from build123d import *

# Parameters (mm, degrees)
F0_R     = 12.7
F1_DEPTH = 25.4
F2_W     = 88.9
F2_H     = 50.8
F3_DEPTH = 50.8
F5_DEPTH = 88.9
F7_DEPTH = 75.946
F8_R     = 12.7
F9_DEPTH = 112.776


# Not quite as in the source:
# - a feature names something its author has since deleted; it is built from what else it names


with BuildPart() as f1:
    # F0 (on Top) → F1 (new body)
    with BuildSketch(Plane.XY):
        with BuildLine():
            Line((-63.5, -31.75), (63.5, -31.75))
            ThreePointArc((63.5, -31.75), (95.25, 0), (63.5, 31.75))
            Line((63.5, 31.75), (-63.5, 31.75))
            ThreePointArc((-63.5, 31.75), (-95.25, 0), (-63.5, -31.75))
        make_face()
        with Locations((-63.5, 0)):
            Circle(F0_R, mode=Mode.SUBTRACT)
        with Locations((63.5, 0)):
            Circle(F0_R, mode=Mode.SUBTRACT)
    extrude(amount=F1_DEPTH)

    # F2 (on face) → F3 (join)
    with BuildSketch(Plane.XY.offset(25.4)):
        Rectangle(F2_W, F2_H)
    extrude(amount=F3_DEPTH)

    # F4 (on face) → F5 (join)
    with BuildSketch(Plane(origin=(-44.45, 0, 0), x_dir=(0, -1, 0), z_dir=(-1, 0, 0))):
        with BuildLine():
            Line((-25.4, 76.2), (25.4, 76.2))
            ThreePointArc((25.4, 76.2), (0, 101.6), (-25.4, 76.2))
        make_face()
    extrude(amount=-F5_DEPTH)

    # F6 (on face) → F7 (cut)
    with BuildSketch(Plane.XZ.offset(25.4)):
        with BuildLine():
            Line((-30.48, 76.2), (30.48, 76.2))
            ThreePointArc((30.48, 76.2), (0, 106.68), (-30.48, 76.2))
        make_face()
        with BuildLine():
            ThreePointArc((-30.48, 76.2), (0, 45.72), (30.48, 76.2))
            Line((30.48, 76.2), (-30.48, 76.2))
        make_face()
        with BuildLine():
            Line((30.48, 76.2), (30.48, 114.3))
            Line((30.48, 114.3), (-30.48, 114.3))
            Line((-30.48, 114.3), (-30.48, 76.2))
            ThreePointArc((-30.48, 76.2), (0, 106.68), (30.48, 76.2))
        make_face()
    extrude(amount=-F7_DEPTH, mode=Mode.SUBTRACT)

    # F8 (on face) → F9 (cut)
    with BuildSketch(Plane(origin=(-44.45, 0, 0), x_dir=(0, -1, 0), z_dir=(-1, 0, 0))):
        with Locations((0, 76.2)):
            Circle(F8_R)
    extrude(amount=-F9_DEPTH, mode=Mode.SUBTRACT)


solid = f1.part
Input: part model. Units: mm. Frame: model coordinates. A direction names the side the tool comes from. Coordinates: 2 decimals unless noted, no trailing zeros. Loops run counter-clockwise (first coordinate to the right, second up) from the corner with the lowest first, then second, coordinate; pieces in that order, holes last.
(1) Section A-A on x = 0. Return the cut outline in (y, z).
(2) Set-up query: faces 1 (the face through (-1, -25.4, 45)), 2 (the face through (44.45, 0, 56)), 3 (the face through (-44.45, 0, 56)), 4 (the face through (-1, 25.4, 45)), 5 (the face through (-30.48, -0.4, 89.1)). Return all of +Z, -Z, +X, -X, +Y, -Y with unobstructed straight access to the full face (end or side cutting, diameter ignored); none if empty.
(3) Section D-D on z = 94. Return the cut outline in (x, y), then the cut area to 3 significant figures.
(4) Material intervals for probe 1 along Y at (x, z) = (63.5, 17); probe 2 along Y at (x, z) = (63, 6); probe 3 along X at (y, z) = (-13.5, 44.5), sorted ascending.
(5) Pull-direction query (X, two-part tool) for faces 6 (the face through (75.614, 3.815, 12.522)), 7 (the face through (-1, -31.75, 13)), 8 (the face through (-95.242, 0.698, 12.522)); classes: released by +X, released by -X, zero draft, split by the parting line, or undercut.
(6) Section C-C on y = 0. Return the cut outline in (x, z).
(7) Section B-B on z = 10.5. Return the cut outline in (x, y).
(8) First-contact query: pin 1 Ø7.5 at (y, z) = (1.5, 90.5) entering from -X; pin 2 Ø12 at (y, z) = (-23.5, 15.5) entering from +X; pin 3 Ø2 at (x, z) = (39.5, 39.5) entering from +Y. Flat tips, straight axial feed; report the tip coordinate or a pass-through.
Data:
1. outline: (-31.75, 0) - (31.75, 0) - (31.75, 25.4) - (25.4, 25.4) - (25.4, 45.72) - (-25.4, 45.72) - (-25.4, 25.4) - (-31.75, 25.4) - close
2. face 1: +Z, +X, -X, -Y
2. face 2: +Z, +X, +Y, -Y
2. face 3: +Z, -X, +Y, -Y
2. face 4: +Z, +X, -X, +Y
2. face 5: +Z, +Y, -Y
3. outline: (-44.45, -18.12) - (-30.48, -18.12) - (-30.48, 18.12) - (-44.45, 18.12) - close; (30.48, -18.12) - (44.45, -18.12) - (44.45, 18.12) - (30.48, 18.12) - close
3. area: 1,010 mm2
4. probe 1: y = -31.75 to -12.7, 12.7 to 31.75
4. probe 2: y = -31.75 to -12.69, 12.69 to 31.75
4. probe 3: x = -44.45 to 44.45
5. face 6: undercut
5. face 7: zero draft
5. face 8: released by -X
6. outline: (-95.25, 0) - (-76.2, 0) - (-76.2, 25.4) - (-95.25, 25.4) - close; (-50.8, 0) - (50.8, 0) - (50.8, 25.4) - (44.45, 25.4) - (44.45, 63.5) - (27.71, 63.5) arc R30.48 cw to (-27.71, 63.5) - (-44.45, 63.5) - (-44.45, 25.4) - (-50.8, 25.4) - close; (-44.45, 88.9) - (-30.48, 88.9) - (-30.48, 101.6) - (-44.45, 101.6) - close; (30.48, 88.9) - (44.45, 88.9) - (44.45, 101.6) - (30.48, 101.6) - close; (76.2, 0) - (95.25, 0) - (95.25, 25.4) - (76.2, 25.4) - close
7. outline: (-63.5, -31.75) - (63.5, -31.75) arc R31.75 ccw to (63.5, 31.75) - (-63.5, 31.75) arc R31.75 ccw to start; hole circle Ø25.4 at (-63.5, 0); hole circle Ø25.4 at (63.5, 0)
8. pin 1: stops at x = -44.45
8. pin 2: stops at x = 89.99
8. pin 3: stops at y = 25.4
